```python
from build123d import *

# Parameters (mm, degrees)
F0_W     = 19.05
F0_H     = 38.6983451158
F0_H_2   = 127
F0_H_3   = 1.5088043451
F1_DEPTH = 38.1


with BuildPart() as f1:
    # F0 (on Front) → F1 (new body)
    with BuildSketch(Plane.XZ):
        Polygon((82.55, -83.5251413941), (19.05, -83.5251413941), (19.05, -85.0339457393), (0, -85.0339457393), (0, -108.9251413941), (82.55, -108.9251413941), align=None)
        Polygon((0, -44.8267962784), (0, -6.7267962784), (-19.05, -6.7267962784), (-82.55, -6.7267962784), (-82.55, -44.8267962784), (-19.05, -44.8267962784), align=None)
        Polygon((19.05, -6.7267962784), (0, -6.7267962784), (0, -44.8267962784), (19.05, -44.8267962784), (82.55, -44.8267962784), (82.55, -6.7267962784), align=None)
        with Locations((9.525, -64.1759688362)):
            Rectangle(F0_W, F0_H)
        with Locations((-9.525, -64.1759688362)):
            Rectangle(F0_W, F0_H)
        with Locations((9.525, 56.7732037216)):
            Rectangle(F0_W, F0_H_2)
        Polygon((0, -85.0339457393), (0, -83.5251413941), (-19.05, -83.5251413941), (-82.55, -83.5251413941), (-82.55, -108.9251413941), (0, -108.9251413941), align=None)
        with Locations((-9.525, 56.7732037216)):
            Rectangle(F0_W, F0_H_2)
        with Locations((9.525, -84.2795435667)):
            Rectangle(F0_W, F0_H_3)
    extrude(amount=F1_DEPTH)


solid = f1.part
```
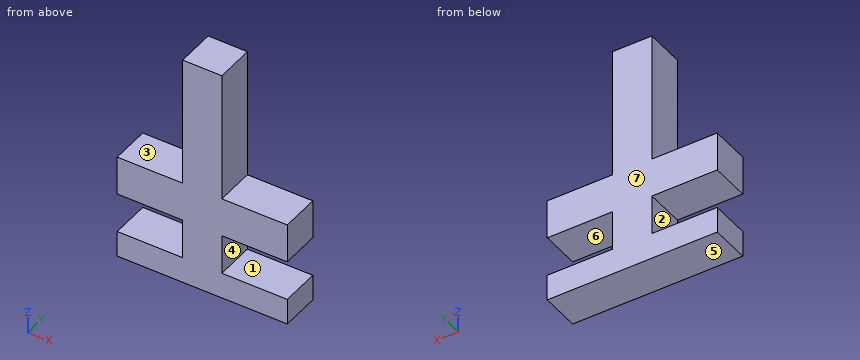
Part model, mm, in its own coordinate system. Face numbers are marked on the shaded views. A direction names the side the tool comes from. Round coordinates to 2 decimals unless told otherwise and drop trailing zeros. Order: outer loops, then holes, each group sorted by start corner. A loop starts at its lowest first (then second) coordinate and runs counter-clockwise, first axis right, second up. Notation, with made-up numbers: M 64.5,48.5 L 83.5,48.5 A5 ccw 83.5,55.5 Z; hole C -29,6 d6. An arc over 180 degrees is marked long. Answer in a Markdown table with one row per item. Add a question column.
Q1. Cut at B-B on y = -23.5. Give the cut face in (x, z).
Q2. Cut at C-C on z = 53. Give the cut face in (x, y).
Q3. Mould opens along Z. For the marked faces 4, 5, 6 and 7 say: +Z half, -Z half, draft (parallel to the pull), parting line (faces both ways), or undercut.
Q4. 3-axis set-ups, long thin cutter, end or side, ignore diameter. For the marked faces 1, 2 and 3: which of +Z, -Z, +X, -X, +Y, -Y reach the whole face in a straight line?
Q5. Pin check, flat tips, straight feed: pin 1 (8 mm diameter, centred on y = -22, z = 1, fed in from -X); pin 2 (1 mm diameter, centred on y = -34, z = 57, fed in from +X); pin 3 (2 mm diameter, centred on x = -60.5, y = -6.5, fed in from +Z). Stop position of each tip, or through.
Q6. Wall check: L1, parallel to Z at x = 60.5, y = -33; L2, parallel to X at y = -3, z = 79. Give the ranges that are in metal, low to high. Write a range as from..to.
Q7. Cut at A-A on x = 55. Give the cut face in (y, z), and give its area (3 significant figures).
Established:
| question | item | result |
|---|---|---|
| 1 | outline | M -82.55,-108.93 L 82.55,-108.93 L 82.55,-83.53 L 19.05,-83.53 L 19.05,-44.83 L 82.55,-44.83 L 82.55,-6.73 L 19.05,-6.73 L 19.05,120.27 L -19.05,120.27 L -19.05,-6.73 L -82.55,-6.73 L -82.55,-44.83 L -19.05,-44.83 L -19.05,-83.53 L -82.55,-83.53 Z |
| 2 | outline | M -19.05,-38.1 L 19.05,-38.1 L 19.05,0 L -19.05,0 Z |
| 3 | face 4 | undercut |
| 3 | face 5 | -Z half |
| 3 | face 6 | undercut |
| 3 | face 7 | draft |
| 4 | face 1 | +X, +Y, -Y |
| 4 | face 2 | -X, +Y, -Y |
| 4 | face 3 | +Z, -X, +Y, -Y |
| 5 | pin 1 | stops at x = -19.05 |
| 5 | pin 2 | stops at x = 19.05 |
| 5 | pin 3 | stops at z = -6.73 |
| 6 | L1 | z = -108.93..-83.53, -44.83..-6.73 |
| 6 | L2 | x = -19.05..19.05 |
| 7 | outline | M -38.1,-108.93 L 0,-108.93 L 0,-83.53 L -38.1,-83.53 Z; M -38.1,-44.83 L 0,-44.83 L 0,-6.73 L -38.1,-6.73 Z |
| 7 | area | 2,420 mm2 |
